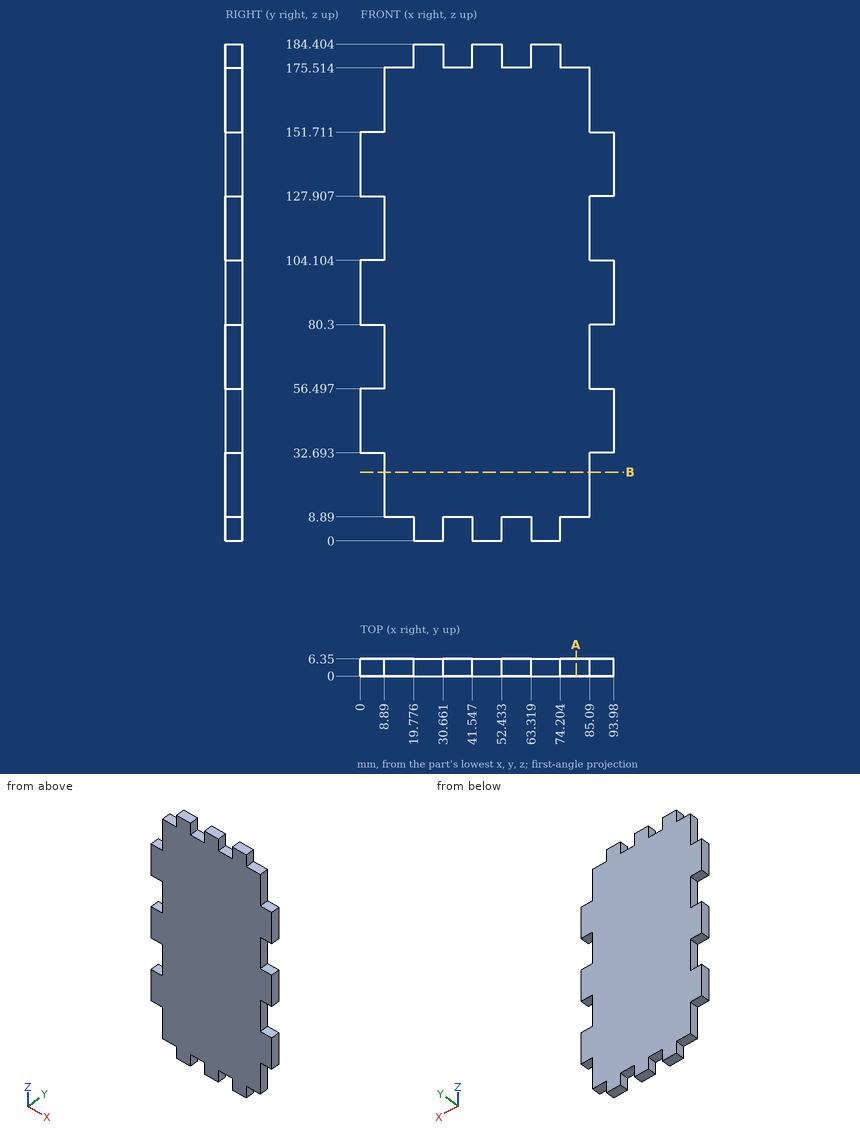
Geometry: see drawing. Coordinates: mm, zero at the bounding-box minimum. Round coordinates to 2 decimals unless told otherwise and drop trailing zeros. Order: outer loops, then holes, each group sorted by start corner. A loop starts at its lowest first (then second) coordinate and runs counter-clockwise, first axis right, second up. Notation, with made-up numbers: (41.25, -31.5) - (84.25, -31.5) arc R14 cw to (84.25, -12.5) - close; hole circle Ø11 at (47.5, -7.5). An arc over 180 degrees is marked (long way). Use a Markdown table: item, result. Add a question column.
1. Section query A-A (x = 80). Return the cut outline in (y, z).
2. Line query: probe 1 along Z at (x, y) = (6, 2); probe 2 along X at (y, z) = (5.75, 176.5) (1 decimal); probe 3 along Z at (x, y) = (59.5, 2.75). Output: solid intervals per line, ascending.
3. First-contact query: pin 1 (1.9 mm diameter, centred on y = 3, z = 3, fed in from +X); pin 2 (3 mm diameter, centred on x = 79, y = 3, fed in from +Z); pin 3 (3 mm diameter, centred on x = 4.5, y = 2.5, fed in from -Z). Flat tips, straight axial feed; report the tip coordinate or a pass-through.
4. Section query B-B (z = 25.5). Return the cut outline in (x, y), then the cut area to 3 significant figures.
Derived:
| question | item | result |
|---|---|---|
| 1 | outline | (0, 8.89) - (6.35, 8.89) - (6.35, 175.51) - (0, 175.51) - close |
| 2 | probe 1 | 32.69 to 56.5, 80.3 to 104.1, 127.91 to 151.71 |
| 2 | probe 2 | 19.8 to 30.7, 41.5 to 52.4, 63.3 to 74.2 |
| 2 | probe 3 | 8.89 to 175.51 |
| 3 | pin 1 | x = 74.2 |
| 3 | pin 2 | z = 175.51 |
| 3 | pin 3 | z = 32.69 |
| 4 | outline | (8.89, 0) - (85.09, 0) - (85.09, 6.35) - (8.89, 6.35) - close |
| 4 | area | 484 mm2 |
